Geometry: final body of the model. Coordinates: model frame, mm. A direction names the side the tool comes from. Give positions to 0.01 mm unless a question says otherwise; leave off trailing zeros. Answer in a Markdown table with one row per item. Add a question column.
Q1. Cut plane A-A on y = 0. Count the separate pieces of the cut face and the enclosed holes in it, and give its area (3 significant figures).
Q2. Line query: line 1 along Y through (x, z) = (47.5, 35); line 2 along X through (y, z) = (-45, 65); line 3 along X through (y, z) = (45, 66.25). Output: solid intervals per line, ascending. Write a range as from..to.
Q3. Pull-direction query (Z, two-part tool) for faces 1 (the face through (0, 48, 70)), 2 (the face through (50, -1, 42)), 3 (the face through (-48.262, -0.651, 39.957)); classes: +Z half, -Z half, draft (parallel to the pull), parting line (faces both ways), or undercut.
Q4. Set-up query: faces 4 (the face through (-1, 0, 5)), 5 (the face through (-42.973, 46.859, 63.916)), 6 (the face through (-50, -1, 42)). Return all of +Z, -Z, +X, -X, +Y, -Y with unobstructed straight access to the full face (end or side cutting, diameter ignored); none if empty.
Q5. Contact query for flat-ended pins moving along their axis: P1, Ø1, axis at x = 21.5, y = 13.5, coming from the +Z side; P2, Ø4.5, axis at x = -45, y = 45, coming from the +Z side. Output: stop coordinate, or through.
from build123d import *

# Parameters (mm, degrees)
F0_W       = 100
F0_H       = 100
F1_DEPTH   = 70
F2_W       = 90
F2_H       = 90
F3_DEPTH   = 65
F3_TAPER   = -3
F4_R       = 5
F1_FACE2_W = 100
F1_FACE2_H = 70
F5_DEPTH   = 100.001
F6_SIZE    = 10
F7_D       = 5.5
F7_DEPTH   = 12
F7_TIP     = 1.6523667023


with BuildPart() as f1:
    # F0 (on Top) → F1 (new body)
    with BuildSketch(Plane.XY):
        Rectangle(F0_W, F0_H)
    extrude(amount=F1_DEPTH)

    # F2 (on face) → F3 (cut)
    with BuildSketch(Plane.XY.offset(70)):
        Rectangle(F2_W, F2_H)
    extrude(amount=-F3_DEPTH, taper=F3_TAPER, mode=Mode.SUBTRACT)

    # F4 (on face) + F1_face2 (on face) → F5 (cut, through all)
    with BuildSketch(Plane.YZ.offset(50)):
        with Locations((0, 35)):
            Circle(F4_R)
    with BuildSketch(Plane(origin=(-50, 0, 35), x_dir=(0, -1, 0), z_dir=(-1, 0, 0))):
        Rectangle(F1_FACE2_W, F1_FACE2_H)
    extrude(amount=-F5_DEPTH, dir=(1, 0, 0), mode=Mode.SUBTRACT)

    # F6
    f6_edges = [f1.edges().sort_by_distance(p)[0] for p in [
        (46.703253, 46.703253, 37.5),
        (-46.703253, 46.703253, 37.5),
        (-46.703253, -46.703253, 37.5),
        (46.703253, -46.703253, 37.5),
    ]]
    chamfer(f6_edges, length=F6_SIZE)

    # F7
    with Locations(Plane.XY.offset(70)):
        with Locations((-45, -45), (-45, 45), (45, 45), (45, -45)):
            Hole(F7_D / 2, depth=F7_DEPTH)
            with Locations((0, 0, -(F7_DEPTH + F7_TIP / 2))):  # 118° drill point
                Cone(0, F7_D / 2, F7_TIP, mode=Mode.SUBTRACT)


solid = f1.part
Completed:
| question | item | result |
|---|---|---|
| 1 | separate pieces | 3 |
| 1 | enclosed holes | 0 |
| 1 | area | 865 mm² |
| 2 | line 1 | y = -50..-5, 5..50 |
| 2 | line 2 | x = -50..-47.75, -42.25..-35.51, 35.51..42.25, 47.75..50 |
| 2 | line 3 | x = -50..-47.75, -42.25..-35.38, 35.38..42.25, 47.75..50 |
| 3 | face 1 | +Z half |
| 3 | face 2 | draft |
| 3 | face 3 | undercut |
| 4 | face 4 | none |
| 4 | face 5 | +Z |
| 4 | face 6 | +Z, -Z, -X, +Y, -Y |
| 5 | P1 | stops at z = 5 |
| 5 | P2 | stops at z = 57.7 |
